Check sheet for the drawn part. Datum: minimum x, y, z corner. Units: mm. A direction names the side the tool comes from. Round coordinates to 2 decimals unless told otherwise and drop trailing zeros. Write each loop counter-clockwise with the first axis right and the second up, starting at its lowest first coordinate (ties: lowest second). Pieces come first, ordered by that corner, then holes. Notation, with made-up numbers: M 61,33.25 L 107,33.25 A18 ccw 107,49.25 Z; hole C 19,89 d8. An arc over 180 degrees is marked long. One line per item, written item: value. Start each with the question number.
1. Depth check by flat-ended pin: P1, Ø1.5, axis at x = 2, y = 3.5, coming from the -Z side; P2, Ø4, axis at y = 1.5, z = 9, coming from the -X side; P3, Ø3, axis at y = 3, z = 35, coming from the +X side. Enter the tip coordinate at first touch or a pass-through.
2. Access from +Z, -Z, +X, -X, +Y, -Y to the whole of each face (thin tool, end or side, straight path). Record for the marked faces 1, 2 and 3.
3. Section check D-D (z = 34.5). Record the boundary of the cut face in (x, y), and give its area (3 significant figures).
4. Section check A-A (x = 5). Record the boundary of the cut face in (y, z).
5. Scan lines: probe 1 along Z at (x, y) = (3, 9); probe 2 along Y at (x, z) = (5, 36); probe 3 along Y at (x, z) = (5.75, 33.5). Record each from-to range of solid material in increasing order. Write a range as [from, to].
6. Section check C-C (z = 17.5). Record the boundary of the cut face in (x, y), and give its area (3 significant figures).
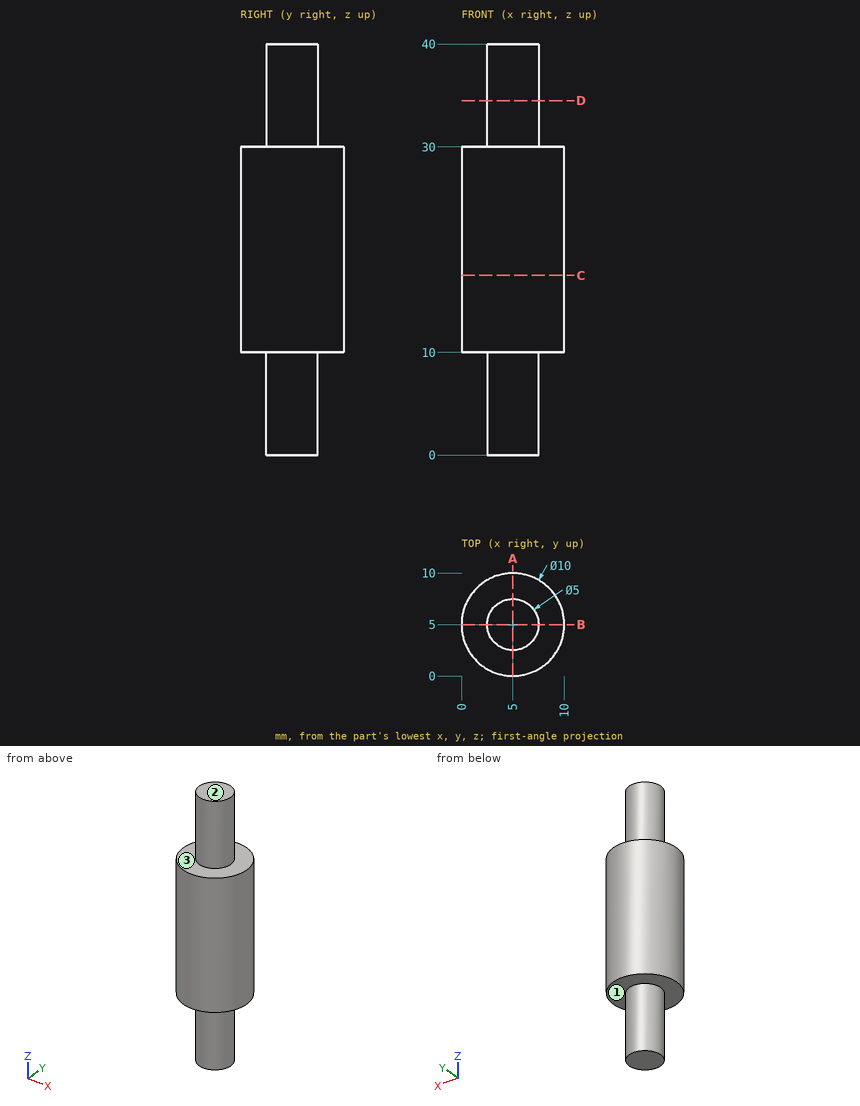
Result sheet:
1. P1: stops at z = 10
1. P2: stops at x = 0.32
1. P3: stops at x = 7.45
2. face 1: -Z
2. face 2: +Z, +X, -X, +Y, -Y
2. face 3: +Z
3. outline: C 5,5 d5
3. area: 19.6 mm2
4. outline: M 0,10 L 2.5,10 L 2.5,0 L 7.5,0 L 7.5,10 L 10,10 L 10,30 L 7.5,30 L 7.5,40 L 2.5,40 L 2.5,30 L 0,30 Z
5. probe 1: z = [10, 30]
5. probe 2: y = [2.5, 7.5]
5. probe 3: y = [2.62, 7.38]
6. outline: C 5,5 d10
6. area: 78.5 mm2
